Autodesk Inventor part; units mm, degrees
ref_plane "YZ Plane" through (0, 0, 0) normal (1, 0, 0) x (0, 1, 0)
ref_plane "XZ Plane" through (0, 0, 0) normal (0, 1, 0) x (-1, 0, 0)
ref_plane "XY Plane" through (0, 0, 0) normal (0, 0, 1) x (1, 0, 0)
sketch "Sketch1" plane through (0, 0, 0) normal (0, 0, 1) x (1, 0, 0)
  line L0 (-32, 27) -> (32, 27)
  line L1 (32, 27) -> (32, -27)
  line L2 (32, -27) -> (-32, -27)
  line L3 (-32, -27) -> (-32, 27)
  line L4 (-32, 27) -> (32, -27) construction
  line L5 (32, 27) -> (-32, -27) construction
  line L6 (35, 30) -> (-35, 30)
  line L7 (-35, 30) -> (-35, -30)
  line L8 (-35, -30) -> (35, -30)
  line L9 (35, -30) -> (35, 30)
  point P0 (0, 0)
  dimension "d0" = 64
  dimension "d1" = 54
  dimension "d2" = 3
extrude "Extrusion1" add sketch "Sketch1" along normal blind 40
sketch "Sketch2" plane through (0, 0, 40) normal (0, 0, 1) x (1, 0, 0)
  line L0 (35, 30) -> (-35, 30)
  line L1 (35, -30) -> (35, 30)
  line L2 (-35, 30) -> (35, 30)
  line L3 (35, 30) -> (35, -30)
  line L4 (35, -30) -> (-35, -30)
  line L5 (-35, -30) -> (-35, 30)
  point P0 (0, 0)
extrude "Extrusion2" add sketch "Sketch2" along normal blind 3
sketch "Sketch3" plane through (35, -30, 0) normal (1, 0, 0) x (0, 0, -1)
  line L0 (0, 3) -> (-27, 3)
  line L1 (-27, 3) -> (-27, 55)
  line L2 (-27, 55) -> (0, 55)
  line L3 (0, 55) -> (0, 3)
  line L4 (0, 3) -> (-27, 55) construction
  line L5 (-27, 3) -> (0, 55) construction
  line L6 (0, 0) -> (0, 60)
  point P0 (0, 30)
  point P1 (-13.5, 29)
  dimension "d7" = 27
  dimension "d8" = 52
  dimension "d9" = 13.5
extrude "Extrusion3" cut sketch "Sketch3" against normal through all
sketch "Sketch4" plane through (-35, -30, 0) normal (0, -1, 0) x (1, 0, 0)
  point P0 (35, 0)
sketch "Sketch5" plane through (0, 0, 0) normal (0, 0, -1) x (-1, 0, 0)
  line L0 (10, -30) -> (-10, -30)
  line L1 (-10, -30) -> (-10, -45)
  line L2 (-10, -45) -> (10, -45)
  line L3 (10, -45) -> (10, -30)
  line L4 (10, -30) -> (-10, -45) construction
  line L5 (-10, -30) -> (10, -45) construction
  line L6 (35, -27) -> (-35, -27)
  point P0 (0, 0)
  point P1 (0, -37.5)
  dimension "d12" = 20
  dimension "d13" = 15
  dimension "d14" = 10.5
extrude "Extrusion4" add sketch "Sketch5" against normal blind 3
ref_plane "Work Plane1" through (-35, -1, 43) normal (0, -1, 0) x (1, 0, 0)
mirror "Mirror1" about plane through (-35, -1, 43) normal (0, -1, 0) of "Extrusion4"
chamfer "Chamfer1" distance 2 angle 45 6 edges at (10, -30, 1.5) (0, -30, 3) (-10, -30, 1.5) (10, 30, 1.5) (0, 30, 3) (-10, 30, 1.5)
fillet "Fillet1" radius 2 8 edges at (10, -45, 1.5) (-10, -45, 1.5) (-35, 0, 43) (0, -30, 43) (35, 0, 43) (0, 30, 43) (10, 43, 1.5) (-10, 43, 1.5)
sketch "Sketch7" plane through (0, 0, 43) normal (0, 0, 1) x (1, 0, 0)
  line L0 (-19, -26) -> (19, -26)
  line L1 (19, -26) -> (19, 26)
  line L2 (19, 26) -> (-19, 26)
  line L3 (-19, 26) -> (-19, -26)
  line L4 (-19, -26) -> (19, 26) construction
  line L5 (19, -26) -> (-19, 26) construction
  point P0 (0, 0)
  dimension "d25" = 38
  dimension "d26" = 52
extrude "Extrusion6" cut sketch "Sketch7" against normal blind 3
sketch "Sketch8" plane through (-10, 32, 3) normal (0, 0, 1) x (1, 0, 0)
  line L0 (2, 11) -> (18, 11)
  line L1 (20, 9) -> (20, 0)
  point P0 (10, -32)
  point P1 (10, 5.5)
  dimension "d29" = 5.5
  dimension "d30" = 10
hole "Hole1" at (0, 37.5, 3) direction (0, 0, -1) diameter 5 end through all
mirror "Mirror2" about plane through (-35, -1, 43) normal (0, -1, 0) of "Hole1"
properties part number "Eletronica - ProtecaoRele"
For this review, take the finished solid that the model builds, in its own axes (mm). A direction names the side the tool comes from. Round coordinates to 2 decimals unless told otherwise and drop trailing zeros. Write each loop counter-clockwise with the first axis right and the second up, starting at its lowest first coordinate (ties: lowest second). Pieces come first, ordered by that corner, then holes. Notation, with made-up numbers: M -18.5,75.25 L 32.5,75.25 A26 cw 32.5,94.25 Z; hole C -10,-23.5 d6. An arc over 180 degrees is marked long. Write item = value, one per line. Start each with the question number.
(1) We need section D-D (z = 33.5). Give the boundary of the cut face in (x, y).
(2) For faces 1 (the face through (0, -26, 42)), 2 (the face through (-10, -38, 1)), 3 (the face through (10, 37, 1)), list the 3-axis set-ups (+Z, -Z, +X, -X, +Y, -Y) from which the entire face can be reached by the end or side of a thin tool; tool diameter is ignored.
(3) We need section C-C (y = -19). Give the boundary of the cut face in (x, z).
(4) We need section B-B (x = 11). Give the boundary of the cut face in (y, z), then the cut area to 3 significant figures.
(5) The part is to be moulded in two halves that separate along X. For faces 4 (the face through (9.43, 42.4, 1.52)), 5 (the face through (0, 43, 1)), 6 (the face through (-22, 0, 40)), say which applies: +X half, -X half, draft (parallel to the pull), parting line (faces both ways), or undercut.
(6) For line 1 along Y through (x, z) = (0, 1); line 2 along Y through (x, z) = (-23, 38); line 3 along X through (y, z) = (-39.5, 1.6), list the stretches that pass through material, from the lowest coordinate up.
(7) We need section A-A (z = 21.5). Give the boundary of the cut face in (x, y), then the cut area to 3 significant figures.
(8) Clearance check with flat-ended pins moving along their axes: pin 1 Ø4 at (x, y) = (28, 2) entering from -Z; pin 2 Ø1 at (x, z) = (12, 37) entering from +Y; pin 3 Ø2.5 at (y, z) = (37.5, 1) entering from +X. State where each tip first meets the part, or that it passes through.
Results found:
q1.outline = M -35,-30 L 35,-30 L 35,30 L -35,30 Z; hole M -32,-27 L 32,-27 L 32,27 L -32,27 Z
q2.face_1 = +Z, -Z
q2.face_2 = +Z, -Z, -X, -Y
q2.face_3 = +Z, -Z, +X, +Y
q3.outline = M -35,27 L -32,27 L -32,40 L -19,40 L -19,43 L -33,43 A2 ccw -35,41 Z; M 19,40 L 32,40 L 32,27 L 35,27 L 35,41 A2 ccw 33,43 L 19,43 Z
q4.outline = M -31,0 L -27,0 L -27,40 L -26,40 L -26,43 L -28,43 A2 ccw -30,41 L -30,5 L -31,4 Z; M 26,40 L 27,40 L 27,0 L 31,0 L 31,4 L 30,5 L 30,41 A2 ccw 28,43 L 26,43 Z
q4.area = 271 mm²
q5.face_4 = +X half
q5.face_5 = draft
q5.face_6 = undercut
q6.line_1 = -45 to -42, -37 to -27, 27 to 35, 40 to 43
q6.line_2 = -30 to -27, 27 to 30
q6.line_3 = -10 to -2.5, 2.5 to 10
q7.outline = M -35,-30 L 35,-30 L 35,-27 L -35,-27 Z; M -35,25 L -32,25 L -32,27 L 32,27 L 32,25 L 35,25 L 35,30 L -35,30 Z
q7.area = 432 mm²
q8.pin_1 = 40
q8.pin_2 = 30
q8.pin_3 = 10
